Autodesk Inventor part; units mm, degrees
ref_plane "YZ Plane" through (0, 0, 0) normal (1, 0, 0) x (0, 1, 0)
ref_plane "XZ Plane" through (0, 0, 0) normal (0, 1, 0) x (-1, 0, 0)
ref_plane "XY Plane" through (0, 0, 0) normal (0, 0, 1) x (1, 0, 0)
sketch "Sketch1" plane through (0, 0, 0) normal (0, 1, 0) x (-1, 0, 0)
  line L0 (2, -0.85) -> (2, -3.75)
  line L1 (-5, 133.15) -> (2, 133.15)
  line L2 (-5, -3.75) -> (-5, 133.15)
  line L3 (2, -0.85) -> (5, -0.85)
  line L4 (5, -0.85) -> (5, 3.15)
  line L5 (5, 3.15) -> (2, 3.15)
  line L6 (2, 30.9) -> (5, 30.9)
  line L7 (5, 30.9) -> (5, 34.9)
  line L8 (5, 34.9) -> (2, 34.9)
  line L9 (2, 62.65) -> (5, 62.65)
  line L10 (5, 62.65) -> (5, 66.65)
  line L11 (5, 66.65) -> (2, 66.65)
  line L12 (2, 94.4) -> (5, 94.4)
  line L13 (5, 94.4) -> (5, 98.4)
  line L14 (5, 98.4) -> (2, 98.4)
  line L15 (2, 3.15) -> (2, 30.9)
  line L16 (2, 34.9) -> (2, 62.65)
  line L17 (2, 66.65) -> (2, 94.4)
  line L18 (2, 126.15) -> (5, 126.15)
  line L19 (5, 126.15) -> (5, 130.15)
  line L20 (5, 130.15) -> (2, 130.15)
  line L21 (2, 98.4) -> (2, 126.15)
  line L22 (2, -0.85) -> (2, -3.75)
  line L23 (2, -3.75) -> (-5, -3.75)
  line L24 (2, 130.15) -> (2, 133.15)
  point P0 (0, 0)
  point P1 (2, 133.15)
  dimension "d35" = 3
  dimension "d36" = 4
  dimension "d46" = 90
  dimension "d52" = 31.75
  dimension "d57" = 2.9
extrude "Extrusion1" add sketch "Sketch1" along normal blind 3
sketch "Sketch4" plane through (0, 3, 0) normal (0, 1, 0) x (1, 0, 0)
  line L0 (1.7141, -13.1698) -> (0.2738, -13.1698)
  line L1 (0.2738, -13.1698) -> (0.2738, -8.8733)
  line L2 (0.2738, -8.8733) -> (-0.6051, -8.8733)
  line L3 (-0.6051, -8.8733) -> (0.9939, -7.2743)
  line L4 (0.9939, -7.2743) -> (2.5929, -8.8733)
  line L5 (1.7141, -13.1698) -> (1.7141, -8.8733)
  line L6 (1.7141, -8.8733) -> (2.5929, -8.8733)
properties part number "steun" material "Wood (Maple)"
Geometry: final body of the model. Coordinates: model frame, mm. A direction names the side the tool comes from. Round coordinates to 2 decimals unless told otherwise and drop trailing zeros. Loops run counter-clockwise (first coordinate to the right, second up) from the corner with the lowest first, then second, coordinate; pieces in that order, holes last. Notation, with made-up numbers: (37.25, 59) -> (81.25, 59) arc R14 ccw to (81.25, 72) -> close; hole circle Ø3 at (34.5, -27.5). An arc over 180 degrees is marked (long way). Write each question's results on one line, items separated by ' | '.
Item 1: Line query: probe 1 along Z at (x, y) = (-4, 0.45); probe 2 along X at (y, z) = (2.7, 22). Output: solid intervals per line, ascending. Write a range as [from, to].
Answers below:
probe 1: z = [-0.85, 3.15], [30.9, 34.9], [62.65, 66.65], [94.4, 98.4], [126.15, 130.15] | probe 2: x = [-2, 5]
Item 2: Cut plane B-B on z = 19. Return the cut outline in (x, y), and give its area (3 significant figures).
Answers below:
outline: (-2, 0) -> (5, 0) -> (5, 3) -> (-2, 3) -> close | area: 21.0 mm²
Item 3: Cut plane A-A on y = 0.65. Return the cut outline in (x, z), and give its area (3 significant figures).
Answers below:
outline: (-5, -0.85) -> (-2, -0.85) -> (-2, -3.75) -> (5, -3.75) -> (5, 133.15) -> (-2, 133.15) -> (-2, 130.15) -> (-5, 130.15) -> (-5, 126.15) -> (-2, 126.15) -> (-2, 98.4) -> (-5, 98.4) -> (-5, 94.4) -> (-2, 94.4) -> (-2, 66.65) -> (-5, 66.65) -> (-5, 62.65) -> (-2, 62.65) -> (-2, 34.9) -> (-5, 34.9) -> (-5, 30.9) -> (-2, 30.9) -> (-2, 3.15) -> (-5, 3.15) -> close | area: 1,020 mm²
Item 4: Pull-direction query (Z, two-part tool) for faces 1 (the face through (-4, 1, 130.15)), 2 (the face through (-3, 1, 62.65)), 3 (the face through (1, 3, 66)); classes: pulls with the +Z half, pulls with the -Z half, needs draft (parallel to the pull), parting line crosses it, or undercut.
Answers below:
face 1: pulls with the +Z half | face 2: undercut | face 3: needs draft
Item 5: Set-up query: faces 4 (the face through (-2, 1, 80)), 5 (the face through (-2, 1, 132)), 6 (the face through (-2, 1, -2)). Return all of +Z, -Z, +X, -X, +Y, -Y with unobstructed straight access to the full face (end or side cutting, diameter ignored); none if empty.
Answers below:
face 4: -X, +Y, -Y | face 5: +Z, -X, +Y, -Y | face 6: -Z, -X, +Y, -Y
Item 6: Pin query (flat end, axial travel): pin 1 Ø1 at (y, z) = (0.5, 20) entering from -X; pin 2 Ø1.5 at (x, y) = (-4, 1) entering from +Z; pin 3 Ø1.5 at (x, y) = (-3, 1.5) entering from -Z. Return the tip coordinate at first contact, or that it passes through.
Answers below:
pin 1: stops at x = -2 | pin 2: stops at z = 130.15 | pin 3: stops at z = -0.85
